```python
from build123d import *

# Parameters (mm, degrees)
BOSS_EXTRUDE1_DEPTH     = 12.7
SKETCH2_W               = 12.7
SKETCH2_H               = 38.133687951
SKETCH2_W_2             = 38.133687951
SKETCH2_H_2             = 12.7
CUT_EXTRUDE1_DEPTH      = 13.7
SKETCH3_R               = 3.429
CUT_EXTRUDE2_DEPTH      = 13.7
F_1_4_CLEARANCE_HOLE2_D = 6.7564
SKETCH8_W               = 674.6875
SKETCH8_H               = 674.6875
CUT_EXTRUDE4_DEPTH      = 13.7
SKETCH10_W              = 0.3175
SKETCH10_H              = 38.1
SKETCH10_W_2            = 38.1
SKETCH10_H_2            = 0.3175
CUT_EXTRUDE5_DEPTH      = 13.7
CUT_EXTRUDE6_DEPTH      = 13.7


with BuildPart() as part:
    # Sketch1 → Boss-Extrude1 (new body)
    with BuildSketch(Plane(origin=(0, 0, 0), x_dir=(1, 0, 0), z_dir=(0, 1, 0))):
        with BuildLine():
            Line((-598.4875, 0), (-674.6875, 0))
            ThreePointArc((-674.6875, 0), (0, 674.6875), (674.6875, 0))
            Line((674.6875, 0), (598.4875, 0))
            ThreePointArc((598.4875, 0), (0, 598.4875), (-598.4875, 0))
        make_face()
    extrude(amount=BOSS_EXTRUDE1_DEPTH)

    # Sketch2 → Cut-Extrude1 (cut, through all)
    with BuildSketch(Plane(origin=(0, 12.7, 0), x_dir=(1, 0, 0), z_dir=(0, 1, 0))):
        with Locations((0, 617.520656025)):
            Rectangle(SKETCH2_W, SKETCH2_H)
        with Locations((617.520656025, 0)):
            Rectangle(SKETCH2_W_2, SKETCH2_H_2)
        with Locations((0, -617.520656025)):
            Rectangle(SKETCH2_W, SKETCH2_H)
        with Locations((-617.520656025, 0)):
            Rectangle(SKETCH2_W_2, SKETCH2_H_2)
    extrude(amount=-CUT_EXTRUDE1_DEPTH, mode=Mode.SUBTRACT)

    # Sketch3 → Cut-Extrude2 (cut, through all)
    with BuildSketch(Plane(origin=(0, 12.7, 0), x_dir=(1, 0, 0), z_dir=(0, 1, 0))):
        with Locations((-6.35, 633.1585)):
            Circle(SKETCH3_R)
        with Locations((-633.1585, 6.35)):
            Circle(SKETCH3_R)
        with Locations((6.35, 633.1585)):
            Circle(SKETCH3_R)
        with Locations((633.1585, 6.35)):
            Circle(SKETCH3_R)
    extrude(amount=-CUT_EXTRUDE2_DEPTH, mode=Mode.SUBTRACT)

    # 1/4 Clearance Hole2 (through all)
    with Locations(Plane(origin=(0, 12.7, 0), x_dir=(1, 0, 0), z_dir=(0, 1, 0))):
        with Locations((-31.75, 642.9375), (-31.75, 611.1875), (-611.1875, 31.75), (-642.9375, 31.75), (-567.596939292, 235.106350216), (-235.106350216, 567.596939292)):
            Hole(F_1_4_CLEARANCE_HOLE2_D / 2)

    # Sketch8 → Cut-Extrude4 (cut, through all)
    with BuildSketch(Plane(origin=(0, 12.7, 0), x_dir=(1, 0, 0), z_dir=(0, 1, 0))):
        with Locations((337.34375, 337.34375)):
            Rectangle(SKETCH8_W, SKETCH8_H)
    extrude(amount=-CUT_EXTRUDE4_DEPTH, mode=Mode.SUBTRACT)

    # Sketch10 → Cut-Extrude5 (cut, through all)
    with BuildSketch(Plane(origin=(0, 12.7, 0), x_dir=(1, 0, 0), z_dir=(0, 1, 0))):
        with Locations((-0.15875, 655.6375)):
            Rectangle(SKETCH10_W, SKETCH10_H)
        with Locations((-655.6375, 0.15875)):
            Rectangle(SKETCH10_W_2, SKETCH10_H_2)
    extrude(amount=-CUT_EXTRUDE5_DEPTH, mode=Mode.SUBTRACT)

    # Sketch13 → Cut-Extrude6 (cut, through all)
    with BuildSketch(Plane(origin=(0, 12.7, 0), x_dir=(1, 0, 0), z_dir=(0, 1, 0))):
        with BuildLine():
            ThreePointArc((-602.990490798, 249.74984277), (-603.400029696, 248.75875888), (-603.807939635, 247.767003434))
            ThreePointArc((-603.807939635, 247.767003434), (-601.965070474, 243.359248479), (-597.55731552, 245.20211764))
            ThreePointArc((-597.55731552, 245.20211764), (-597.153628267, 246.183606427), (-596.748328919, 247.164430609))
            ThreePointArc((-596.748328919, 247.164430609), (-598.576703778, 251.578217629), (-602.990490798, 249.74984277))
        make_face()
        with BuildLine():
            ThreePointArc((-460.745442177, 462.261996567), (-461.504342318, 461.504342318), (-462.261996567, 460.745442177))
            ThreePointArc((-462.261996567, 460.745442177), (-462.254146876, 455.967952369), (-457.476657068, 455.97580206))
            ThreePointArc((-457.476657068, 455.97580206), (-456.726846061, 456.726846061), (-455.97580206, 457.476657068))
            ThreePointArc((-455.97580206, 457.476657068), (-455.967952369, 462.254146876), (-460.745442177, 462.261996567))
        make_face()
        with BuildLine():
            ThreePointArc((-247.767003434, 603.807939635), (-248.75875888, 603.400029696), (-249.74984277, 602.990490798))
            ThreePointArc((-249.74984277, 602.990490798), (-251.578217629, 598.576703778), (-247.164430609, 596.748328919))
            ThreePointArc((-247.164430609, 596.748328919), (-246.183606427, 597.153628267), (-245.20211764, 597.55731552))
            ThreePointArc((-245.20211764, 597.55731552), (-243.359248479, 601.965070474), (-247.767003434, 603.807939635))
        make_face()
    extrude(amount=-CUT_EXTRUDE6_DEPTH, mode=Mode.SUBTRACT)


solid = part.part
```
For this review, take the finished solid that the model builds, in its own axes (mm). Coordinates: 2 decimals unless noted, no trailing zeros. Loops run counter-clockwise (first coordinate to the right, second up) from the corner with the lowest first, then second, coordinate; pieces in that order, holes last.
1. Add section C-C, the plane z = -342.5. Give the boundary of the cut face in (x, y), then the cut area to 3 significant figures.
2. Add section B-B, the plane x = -319.5. Give the boundary of the cut face in (y, z).
3. Insertion check: P1, Ø3, axis at x = -200.5, y = 8, coming from the -Z side; P2, Ø6.5, axis at y = 6.5, z = -610.5, coming from the +X side; P3, Ø9, axis at x = -235.11, z = -567.6, coming from the +Y side; P4, Ø1.8, axis at y = 4, z = -3, coming from the +X side. Each pin has a flat end and moves straight along its axis. Give the tip position at first contact, or say it passes through.
4. Add section A-A, the plane y = 2.25. Count the separate pieces of the cut face and the enclosed holes in it, then the cut area to 3 significant figures.
5. For line 1 (X direction, y = 6.75, z = -31.75); line 2 (Z direction, x = -536.5, y = 3.25), list the stretches that pass through material, from the lowest coordinate up.
Result:
1. outline: (-581.29, 0) - (-490.8, 0) - (-490.8, 12.7) - (-581.29, 12.7) - close
1. area: 1,150 mm2
2. outline: (0, -594.24) - (12.7, -594.24) - (12.7, -506.07) - (0, -506.07) - close
3. P1: stops at z = -644.67
3. P2: stops at x = -6.35
3. P3: stops at y = 12.7
3. P4: stops at x = -636.59
4. separate pieces: 1
4. enclosed holes: 9
4. area: 75,300 mm2
5. line 1: x = -673.94 to -646.32, -639.56 to -614.57, -607.81 to -597.64
5. line 2: z = -409.11 to -265.25
